Drawing for the job (mm, zero at the part's lowest x, y, z). A direction names the side the tool comes from. Give positions to 0.01 mm unless a question says otherwise; leave off trailing zeros. Write each loop counter-clockwise with the first axis right and the second up, starting at its lowest first coordinate (ties: lowest second). Pieces come first, ordered by that corner, then holes.
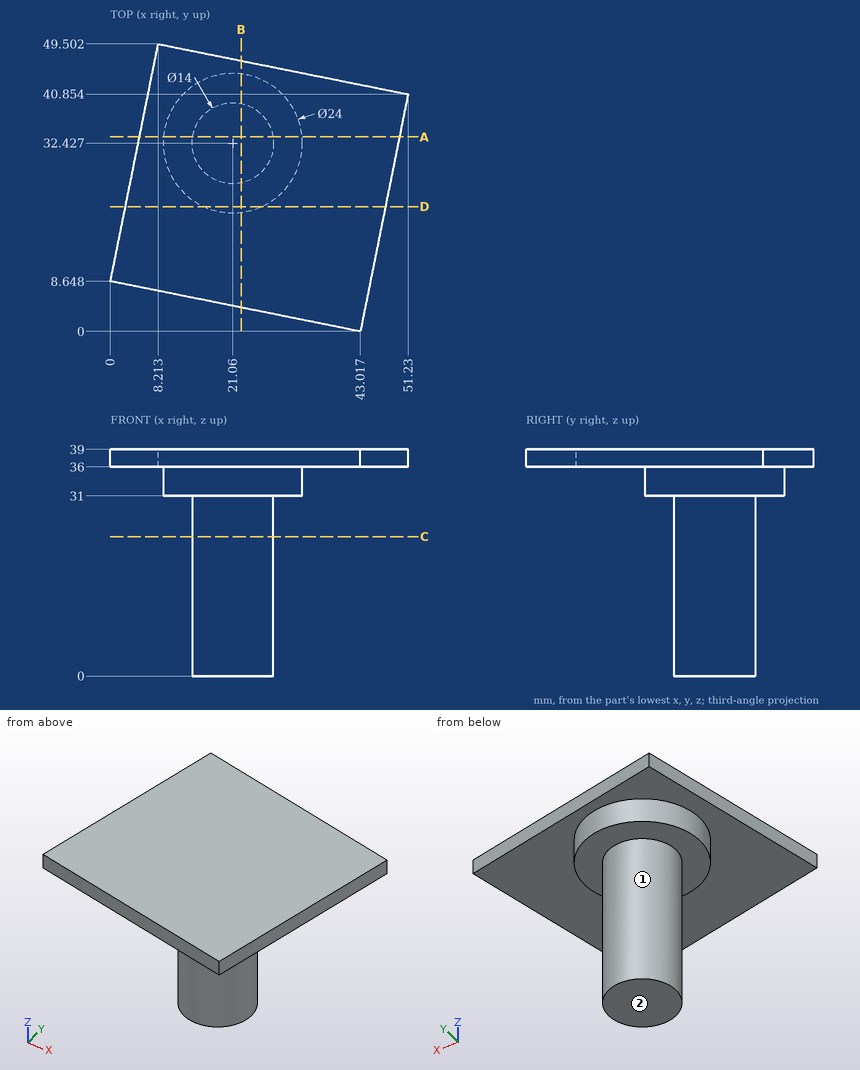
1. Slice it at C-C, the plane z = 24. Write the cut outline in (x, y), and give its area (3 significant figures).
Calculated:
outline: circle Ø14 at (21.06, 32.43)
area: 154 mm2
2. Probe probe 1 along Z at (x, y) = (16, 43); probe 2 along Y at (x, z) = (21, 25); probe 3 along Z at (x, y) = (40.5, 42). List the from-to ranges inside material, lowest first.
Calculated:
probe 1: z = 31 to 39
probe 2: y = 25.43 to 39.43
probe 3: z = 36 to 39
3. Slice it at A-A, the plane y = 33.5. Write the cut outline in (x, z).
Calculated:
outline: (5, 36) - (9.11, 36) - (9.11, 31) - (14.14, 31) - (14.14, 0) - (27.98, 0) - (27.98, 31) - (33.01, 31) - (33.01, 36) - (49.75, 36) - (49.75, 39) - (5, 39) - close
4. Pin check, flat tips, straight feed: P1, Ø12, axis at y = 14, z = 31.5, coming from the -X side; P2, Ø4, axis at x = 30, y = 42, coming from the -Z side; P3, Ø15, axis at x = 37, y = 17, coming from the -Z side. Stop position of each tip, or through.
Calculated:
P1: stops at x = 0.28
P2: stops at z = 31
P3: stops at z = 36
5. Slice it at D-D, the plane y = 21.5. Write the cut outline in (x, z), and give its area (3 significant figures).
Calculated:
outline: (2.58, 36) - (16.1, 36) - (16.1, 31) - (26.02, 31) - (26.02, 36) - (47.34, 36) - (47.34, 39) - (2.58, 39) - close
area: 184 mm2
6. Which spindle directions (+Z, -Z, +X, -X, +Y, -Y) get a long thin tool onto all of the face, cutting with end or side? Do the marked faces 1 and 2. Say none if no direction does.
Calculated:
face 1: -Z
face 2: -Z, +X, -X, +Y, -Y
7. Slice it at B-B, the plane x = 22.5. Write the cut outline in (y, z) (1 decimal).
Calculated:
outline: (4.1, 36) - (20.5, 36) - (20.5, 31) - (25.6, 31) - (25.6, 0) - (39.3, 0) - (39.3, 31) - (44.3, 31) - (44.3, 36) - (46.6, 36) - (46.6, 39) - (4.1, 39) - close
